from build123d import *

# Parameters (mm, degrees)
SKETCH1_W           = 3.959797974
SKETCH1_H           = 3.959797974
BOSS_EXTRUDE1_DEPTH = 6.35
SKETCH2_W           = 15
SKETCH2_H           = 8
BOSS_EXTRUDE2_DEPTH = 44.45
SKETCH3_R           = 6
CUT_EXTRUDE1_DEPTH  = 25.4
SKETCH4_W           = 4.064
SKETCH4_H           = 4.064
BOSS_EXTRUDE3_DEPTH = 20.32
SKETCH5_W           = 8
SKETCH5_H           = 6.35
BOSS_EXTRUDE4_DEPTH = 12.7
SKETCH6_W           = 6.812329396
SKETCH6_H           = 8
BOSS_EXTRUDE5_DEPTH = 6.35


with BuildPart() as part:
    # Sketch1 → Boss-Extrude1 (new body)
    with BuildSketch(Plane(origin=(0, 0, 0), x_dir=(1, 0, 0), z_dir=(0, 1, 0))):
        Rectangle(SKETCH1_W, SKETCH1_H)
    extrude(amount=BOSS_EXTRUDE1_DEPTH)

    # Sketch2 → Boss-Extrude2 (add)
    with BuildSketch(Plane(origin=(0, 6.35, 0), x_dir=(1, 0, 0), z_dir=(0, 1, 0))):
        Rectangle(SKETCH2_W, SKETCH2_H)
    extrude(amount=BOSS_EXTRUDE2_DEPTH)

    # Sketch3 → Cut-Extrude1 (cut)
    with BuildSketch(Plane.XY.offset(4)):
        with Locations((0, 21.59)):
            Circle(SKETCH3_R)
    extrude(amount=-CUT_EXTRUDE1_DEPTH, mode=Mode.SUBTRACT)

    # Sketch4 → Boss-Extrude3 (add)
    with BuildSketch(Plane(origin=(0, 50.8, 0), x_dir=(1, 0, 0), z_dir=(0, 1, 0))):
        Rectangle(SKETCH4_W, SKETCH4_H)
    extrude(amount=BOSS_EXTRUDE3_DEPTH)

    # Sketch5 → Boss-Extrude4 (add)
    with BuildSketch(Plane.ZY.offset(7.5)):
        with Locations((0, 24.765)):
            Rectangle(SKETCH5_W, SKETCH5_H)
    extrude(amount=BOSS_EXTRUDE4_DEPTH)

    # Sketch6 → Boss-Extrude5 (add)
    with BuildSketch(Plane(origin=(0, 27.94, 0), x_dir=(1, 0, 0), z_dir=(0, 1, 0))):
        with Locations((-16.793835302, 0)):
            Rectangle(SKETCH6_W, SKETCH6_H)
    extrude(amount=BOSS_EXTRUDE5_DEPTH)


solid = part.part
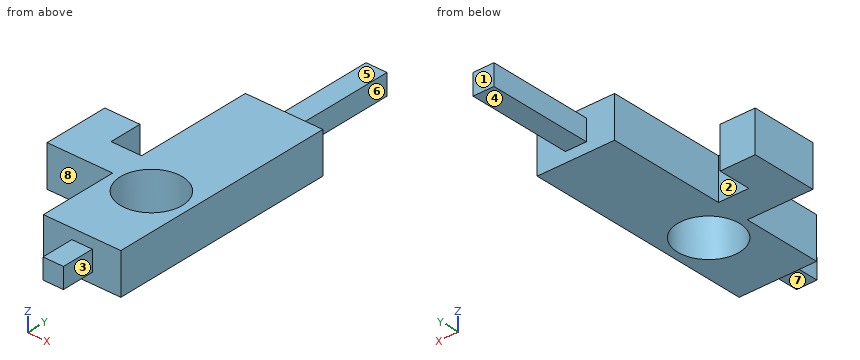
Geometry check sheet. Reference: the model listing, model coordinates, mm. Face numbers are marked on the shaded views. A direction names the side the tool comes from. Round coordinates to 2 decimals unless told otherwise and drop trailing zeros. Loops run counter-clockwise (first coordinate to the right, second up) from the corner with the lowest first, then second, coordinate; pieces in that order, holes last. Notation, with made-up numbers: (76.25, 49) - (106.25, 49) arc R30 ccw to (106.25, 80) - close; hole circle Ø11 at (-30, -39). An arc over 180 degrees is marked (long way). Answer as CSV lines item,"result".
(1) Cross-section at A-A, the plane z = 0.5. Enter the section's corners in (x, y).
Output values:
outline,"(-20.2, 21.59) - (-7.5, 21.59) - (-7.5, 6.35) - (-1.98, 6.35) - (-1.98, 0) - (1.98, 0) - (1.98, 6.35) - (7.5, 6.35) - (7.5, 50.8) - (2.03, 50.8) - (2.03, 71.12) - (-2.03, 71.12) - (-2.03, 50.8) - (-7.5, 50.8) - (-7.5, 27.94) - (-13.39, 27.94) - (-13.39, 34.29) - (-20.2, 34.29) - close; hole circle Ø12 at (0, 21.59)"
(2) Cross-section at C-C, the plane x = -4. Enter the section's corners in (y, z).
Output values:
outline,"(6.35, -4) - (17.12, -4) - (17.12, 4) - (6.35, 4) - close; (26.06, -4) - (50.8, -4) - (50.8, 4) - (26.06, 4) - close"
(3) Cross-section at B-B, the plane x = 0. Enter the section's corners in (y, z), and give its area (3 significant figures).
Output values:
outline,"(0, -1.98) - (6.35, -1.98) - (6.35, -4) - (15.59, -4) - (15.59, 4) - (6.35, 4) - (6.35, 1.98) - (0, 1.98) - close; (27.59, -4) - (50.8, -4) - (50.8, -2.03) - (71.12, -2.03) - (71.12, 2.03) - (50.8, 2.03) - (50.8, 4) - (27.59, 4) - close"
area,"367 mm²"
(4) Cross-section at D-D, the plane y = 36. Enter the section's corners in (x, z), and give its area (3 significant figures).
Output values:
outline,"(-7.5, -4) - (7.5, -4) - (7.5, 4) - (-7.5, 4) - close"
area,"120 mm²"
(5) Material ranges on line 1 along Y through (x, z) = (0, -0.5); line 2 along Y through (x, z) = (-14.5, 3.5); line 3 along Y through (x, z) = (0, 2.25), recorded low to high.
Output values:
line 1,"y = 0 to 15.59, 27.59 to 71.12"
line 2,"y = 21.59 to 34.29"
line 3,"y = 6.35 to 15.59, 27.59 to 50.8"
(6) Release check for a two-part mould opening along X. For the marked faces 1, 2 and 3 record: released by +X, released by -X, zero draft, split by the parting line, or undercut.
Output values:
face 1,"zero draft"
face 2,"undercut"
face 3,"released by +X"
(7) Set-up check for the marked faces 4, 5, 6, 7 and 8: record each of +Z, -Z, +X, -X, +Y, -Y from which the full face is reachable in a straight line by a thin tool's end or side.
Output values:
face 4,"-Z, +X, -X, +Y"
face 5,"+Z, +X, -X, +Y"
face 6,"+Z, -Z, +X, +Y"
face 7,"-Z, +X, -X, -Y"
face 8,"+Z, -Z, -X, -Y"
(8) Depth check by flat-ended pin: pin 1 Ø4.5 at (y, z) = (65, 0) entering from -X; pin 2 Ø4.5 at (y, z) = (62, -1) entering from +X; pin 3 Ø4.5 at (x, y) = (1, 4.5) entering from +Z; pin 4 Ø4 at (y, z) = (16, 0.5) entering from -X. Enter the tip coordinate at first touch or a pass-through.
Output values:
pin 1,"stops at x = -2.03"
pin 2,"stops at x = 2.03"
pin 3,"stops at z = 4"
pin 4,"stops at x = -7.5"
